Input: part model. Units: mm. Frame: model coordinates. A direction names the side the tool comes from. Give positions to 0.01 mm unless a question says otherwise; leave off trailing zeros. Loops run counter-clockwise (first coordinate to the right, second up) from the corner with the lowest first, then second, coordinate; pieces in that order, holes last. Notation, with made-up numbers: (-6.75, -35.5) - (0.25, -35.5) arc R23 cw to (0.25, 2.5) - close; hole circle Ø10 at (21.25, 18.5). An arc over 180 degrees is marked (long way). Answer as a JSON object with one key per item and string values.
from build123d import *

# Parameters (mm, degrees)
BOSS_EXTRUDE1_DEPTH = 40
SKETCH2_W           = 30
SKETCH2_H           = 30
BOSS_EXTRUDE2_DEPTH = 150
BOSS_EXTRUDE4_DEPTH = 30
SKETCH5_R           = 5
CUT_EXTRUDE2_DEPTH  = 30
CIRPATTERN1_COUNT   = 3
SKETCH6_R           = 10
CUT_EXTRUDE3_DEPTH  = 50
SKETCH7_R           = 5
CUT_EXTRUDE4_DEPTH  = 30
SKETCH8_R           = 5
CUT_EXTRUDE5_DEPTH  = 30


with BuildPart() as part:
    # Sketch1 → Boss-Extrude1 (new body)
    with BuildSketch(Plane(origin=(0, 0, 0), x_dir=(1, 0, 0), z_dir=(0, 1, 0))):
        with BuildLine():
            ThreePointArc((-57.082039325, -56.050341538), (0, -80), (57.082039325, -56.050341538))
            ThreePointArc((57.082039325, -56.050341538), (69.282032303, -40), (77.082039325, -21.409325386))
            ThreePointArc((77.082039325, -21.409325386), (79.267153178, -10.80363027), (80, 0))
            ThreePointArc((80, 0), (63.245553203, 48.989794856), (20, 77.459666924))
            ThreePointArc((20, 77.459666924), (0, 80), (-20, 77.459666924))
            ThreePointArc((-20, 77.459666924), (-69.282032303, 40), (-77.082039325, -21.409325386))
            ThreePointArc((-77.082039325, -21.409325386), (-69.282032303, -40), (-57.082039325, -56.050341538))
        make_face()
        with BuildLine():
            ThreePointArc((-20, 77.459666924), (0, 80), (20, 77.459666924))
            Line((20, 77.459666924), (20, 200))
            Line((20, 200), (-20, 200))
            Line((-20, 200), (-20, 77.459666924))
        make_face()
        with BuildLine():
            Line((-163.205080757, -117.320508076), (-57.082039325, -56.050341538))
            ThreePointArc((-57.082039325, -56.050341538), (-69.282032303, -40), (-77.082039325, -21.409325386))
            Line((-77.082039325, -21.409325386), (-183.205080757, -82.679491924))
            Line((-183.205080757, -82.679491924), (-163.205080757, -117.320508076))
        make_face()
        with BuildLine():
            Line((57.082039325, -56.050341538), (163.205080757, -117.320508076))
            Line((163.205080757, -117.320508076), (183.205080757, -82.679491924))
            Line((183.205080757, -82.679491924), (77.082039325, -21.409325386))
            ThreePointArc((77.082039325, -21.409325386), (69.282032303, -40), (57.082039325, -56.050341538))
        make_face()
    extrude(amount=BOSS_EXTRUDE1_DEPTH)

    # Sketch2 → Boss-Extrude2 (add)
    with BuildSketch(Plane.XZ):
        with Locations((0, -180)):
            Rectangle(SKETCH2_W, SKETCH2_H)
    boss_extrude2 = extrude(amount=BOSS_EXTRUDE2_DEPTH)

    # Sketch3 → Boss-Extrude4 (add)
    with BuildSketch(Plane(origin=(15, 0, 0), x_dir=(0, 0, -1), z_dir=(1, 0, 0))):
        with BuildLine():
            Line((165, -150), (195, -150))
            ThreePointArc((195, -150), (180, -165), (165, -150))
        make_face()
    boss_extrude4 = extrude(amount=-BOSS_EXTRUDE4_DEPTH)

    # Sketch5 → Cut-Extrude2 (cut)
    with BuildSketch(Plane(origin=(15, 0, 0), x_dir=(0, 0, -1), z_dir=(1, 0, 0))):
        with Locations((180, -150)):
            Circle(SKETCH5_R)
    extrude(amount=-CUT_EXTRUDE2_DEPTH, mode=Mode.SUBTRACT)

    # CirPattern1: Boss-Extrude2, Boss-Extrude4 ×3 about axis
    cirpattern1_axis = Axis((0, 0, 0), (0, 1, 0))
    add([boss_extrude2.rotate(cirpattern1_axis, i * 360 / CIRPATTERN1_COUNT) for i in range(1, CIRPATTERN1_COUNT)])
    add([boss_extrude4.rotate(cirpattern1_axis, i * 360 / CIRPATTERN1_COUNT) for i in range(1, CIRPATTERN1_COUNT)])

    # Sketch6 → Cut-Extrude3 (cut)
    with BuildSketch(Plane(origin=(0, 40, 0), x_dir=(1, 0, 0), z_dir=(0, 1, 0))):
        with Locations(Location((0, 0, 0), (0, 0, 270))):
            Circle(SKETCH6_R)
    extrude(amount=-CUT_EXTRUDE3_DEPTH, mode=Mode.SUBTRACT)

    # Sketch7 → Cut-Extrude4 (cut)
    with BuildSketch(Plane(origin=(7.5, 0, 12.990381057), x_dir=(0.8660254037844434, 0, -0.49999999999999195), z_dir=(0.49999999999999195, 0, 0.8660254037844434))):
        with Locations((-180, -150)):
            Circle(SKETCH7_R)
    extrude(amount=-CUT_EXTRUDE4_DEPTH, mode=Mode.SUBTRACT)

    # Sketch8 → Cut-Extrude5 (cut)
    with BuildSketch(Plane(origin=(-7.5, 0, 12.990381057), x_dir=(0.8660254037844364, 0, 0.5000000000000041), z_dir=(-0.500000000000004, 0, 0.8660254037844363))):
        with Locations((180, -150)):
            Circle(SKETCH8_R)
    extrude(amount=-CUT_EXTRUDE5_DEPTH, mode=Mode.SUBTRACT)


solid = part.part
Item 1: Access query for faces 5 (the face through (168.98, -73.95, 97.32)), 6 (the face through (148.566, -81.345, 103.095)), 7 (the face through (-20, 20, -140)), 8 (the face through (-142.79, -73.95, 82.68)). Directions: +Z, -Z, +X, -X, +Y, -Y. A direction counts if a zero-diameter tool reaches every point of the face in a straight line with its end or side. Return the directions, or none.
Geometry check:
{"face 5": "+Z, +X, -Y", "face 6": "+Z, -Y", "face 7": "-Z, -X, +Y, -Y", "face 8": "-Z, -Y"}
Item 2: Contact query for flat-ended pins moving along their axis: P1, Ø3, axis at y = -2.5, z = -103, coming from the +X side; P2, Ø4, axis at x = 73.5, z = 60, coming from the -Y side; P3, Ø24, axis at y = -68, z = -178, coming from the -X side; P4, Ø15, axis at x = -6.5, y = -38, coming from the +Z side. Output: stop coordinate, or through.
Geometry check:
{"P1": "passes through", "P2": "stops at y = 0", "P3": "stops at x = -15", "P4": "stops at z = -165"}
Item 3: Cut plane D-D (x = 104). Return loops of the section in (y, z).
Geometry check:
{"outline": "(0, 36.95) - (40, 36.95) - (40, 83.14) - (0, 83.14) - close"}
Item 4: Cut plane A-A (x = 0). Return loops of the section in (y, z), then the cut area to 3 significant figures.
Geometry check:
{"outline": "(-150, -195) - (0, -195) - (0, -200) - (40, -200) - (40, -10) - (0, -10) - (0, -165) - (-150, -165) arc R15 ccw to start; (0, 10) - (40, 10) - (40, 80) - (0, 80) - close; hole circle Ø10 at (-150, -180)", "area": "15,200 mm2"}
Item 5: Mould query, pull axis Z, two halves, no side actions, for faces 1 (the face through (0, -153, -176)), 2 (the face through (0, -74, -195)), 3 (the face through (-0.89, 19.72, 79.995)), 4 (the face through (13, 0, -7)). Classes: released by +Z, released by -Z, zero draft, split by the parting line, or undercut.
Geometry check:
{"face 1": "undercut", "face 2": "released by -Z", "face 3": "released by +Z", "face 4": "zero draft"}
Item 6: Cut plane C-C (z = -117.5). Return loops of the section in (x, y), then the cut area to 3 significant figures.
Geometry check:
{"outline": "(-20, 0) - (20, 0) - (20, 40) - (-20, 40) - close", "area": "1,600 mm2"}
Item 7: Material intervals for line 1 (X direction, y = 21, z = 0); line 2 (X direction, y = 19, z = 62); line 3 (Y direction, x = -20.5, z = -43.5), sorted ascending. Write a range as [from, to].
Geometry check:
{"line 1": "x = [-80, -10], [10, 80]", "line 2": "x = [-147.39, -67.39], [-50.56, 50.56], [67.39, 147.39]", "line 3": "y = [0, 40]"}
Item 8: Cut plane B-B (y = -29.5). Return loops of the section in (x, z).
Geometry check:
{"outline": "(-176.37, 84.51) - (-150.39, 69.51) - (-135.39, 95.49) - (-161.37, 110.49) - close; (-15, -195) - (15, -195) - (15, -165) - (-15, -165) - close; (135.39, 95.49) - (150.39, 69.51) - (176.37, 84.51) - (161.37, 110.49) - close"}
